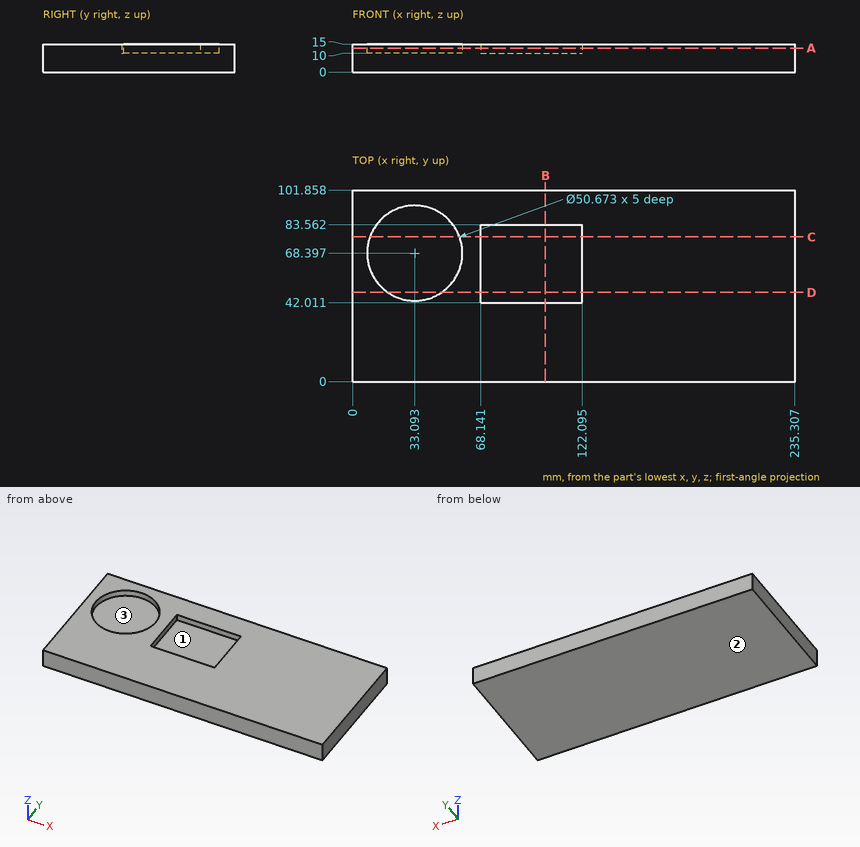
The drawing under review shows one solid part. Ordinate dimensions are in mm from its lowest x, y, z. Coordinates: 2 decimals unless noted, no trailing zeros. Write each loop counter-clockwise with the first axis right and the second up, starting at its lowest first coordinate (ties: lowest second). Pieces come first, ordered by that corner, then holes. Notation, with made-up numbers: (37.25, 43) - (96.25, 43) arc R22 cw to (96.25, 61) - close; hole circle Ø2 at (80, 18.5). An arc over 180 degrees is marked (long way). Answer in a Markdown table with one row per item. Add a question column.
Q1. For P1, Ø1, axis at y = 62.5, z = 7, coming from the -X side; P2, Ø15, axis at x = 45, y = 65, coming from the +Z side, all flat-tipped, find the tip position at first contact; note any pin that passes through.
Q2. We need section A-A, the plane z = 12.75. State the section outline as (x, y) points (1 decimal).
Q3. We need section C-C, the plane y = 77. State the section outline as (x, z) points (1 decimal).
Q4. We need section B-B, the plane x = 102.5. State the section outline as (y, z) points.
Q5. For probe 1 along Y at (x, z) = (81.5, 14); probe 2 along Z at (x, y) = (90.5, 71); probe 3 along Y at (x, z) = (21, 12.25), list the stretches that pass through material, from the lowest coordinate up.
Q6. Draft analysis for pull direction Y (two halves, no side actions). For the marked faces 1, 2 and 3, state which applies: +Y half, -Y half, draft (parallel to the pull), parting line (faces both ways), or undercut.
Q7. We need section D-D, the plane y = 47.5. State the section outline as (x, z) points (1 decimal).
Answer list:
| question | item | result |
|---|---|---|
| 1 | P1 | stops at x = 0 |
| 1 | P2 | stops at z = 10 |
| 2 | outline | (0, 0) - (235.3, 0) - (235.3, 101.9) - (0, 101.9) - close; hole circle Ø50.7 at (33.1, 68.4); hole (68.1, 42) - (122.1, 42) - (122.1, 83.6) - (68.1, 83.6) - close |
| 3 | outline | (0, 0) - (235.3, 0) - (235.3, 15) - (122.1, 15) - (122.1, 10) - (68.1, 10) - (68.1, 15) - (56.9, 15) - (56.9, 10) - (9.3, 10) - (9.3, 15) - (0, 15) - close |
| 4 | outline | (0, 0) - (101.86, 0) - (101.86, 15) - (83.56, 15) - (83.56, 10) - (42.01, 10) - (42.01, 15) - (0, 15) - close |
| 5 | probe 1 | y = 0 to 42.01, 83.56 to 101.86 |
| 5 | probe 2 | z = 0 to 10 |
| 5 | probe 3 | y = 0 to 46.13, 90.66 to 101.86 |
| 6 | face 1 | undercut |
| 6 | face 2 | draft |
| 6 | face 3 | undercut |
| 7 | outline | (0, 0) - (235.3, 0) - (235.3, 15) - (122.1, 15) - (122.1, 10) - (68.1, 10) - (68.1, 15) - (47.4, 15) - (47.4, 10) - (18.8, 10) - (18.8, 15) - (0, 15) - close |
